Input: part model. Units: mm. Frame: model coordinates. A direction names the side the tool comes from. Coordinates: 2 decimals unless noted, no trailing zeros. Write each loop counter-clockwise with the first axis right and the second up, starting at its lowest first coordinate (ties: lowest second). Pieces come first, ordered by that corner, then holes. Notation, with made-up numbers: (-6, 72.25) - (39, 72.25) arc R33 cw to (39, 104.25) - close; hole circle Ø4 at (17.25, 74). An arc over 180 degrees is marked (long way). One line per question, with ' | ' between items. Start each with the question number.
1) First-contact query: P1, Ø1, axis at y = -11, z = 15.5, coming from the -X side; P2, Ø8, axis at x = -27.5, y = -16.5, coming from the -Z side; P3, Ø3.5, axis at x = -32, y = -14.5, coming from the +Z side; P4, Ø10, axis at x = -31, y = 25, coming from the -Z side. Flat tips, straight axial feed; report the tip coordinate or a pass-through.
2) Section query A-A on x = -25. Return loops of the section in (y, z), and give its area (3 significant figures).
3) Section query B-B on y = -15. Return loops of the section in (x, z), and give its area (3 significant figures).
4) Line query: line 1 (X direction, y = -9, z = 19.75); line 2 (X direction, y = 17.5, z = 12); line 3 (X direction, y = -14.5, z = 8.5). Output: solid intervals per line, ascending.
5) Reachability of faces 1 (the flat face through (-30, -15, 7.621)), 2 (the flat face through (-35.132, -15, 13)), 3 (the flat face through (-30, -15, 19.284)), 4 (the flat face through (-22.931, 31, 13)) from +Z, -Z, +X, -X, +Y, -Y: full face, straight path, thin tool, end or side. Return the list, or none.
6) Section query C-C on x = -33.5. Return loops of the section in (y, z).
7) Section query D-D on y = -5. Return loops of the section in (x, z).
```python
from build123d import *

# Parameters (mm, degrees)
F1_DEPTH = 25.4
F3_W     = 10.9566785395
F3_H     = 11.6627290845
F4_DEPTH = 7.1539785713


with BuildPart() as f1:
    # F0 (on Top) → F1 (new body)
    with BuildSketch(Plane.XY):
        with BuildLine():
            Line((-42.3919206649, 8.6023595556), (-42.3919206649, -11.4512224138))
            Line((-42.3919206649, -11.4512224138), (-19.3287206649, -11.4512224138))
            Line((-19.3287206649, -11.4512224138), (-19.3287206649, 8.6023595556))
            add(Edge.make_bspline(
                [(-19.3287206649, 8.6023595556), (-16.323673708, 11.7888919971), (-9.9481352571, 18.5494707236), (-16.0846098572, 27.4246591557), (-19.3287206649, 32.1166146935)],
                knots=[0, 0, 0, 0, 0.4713400446, 1, 1, 1, 1], degree=3))
            Line((-19.3287206649, 32.1166146935), (-22.9309096968, 32.1166146935))
            Line((-22.9309096968, 32.1166146935), (-22.9309096968, 29.055005683))
            ThreePointArc((-22.9309096968, 29.055005683), (-30.8603206649, 11.9618341392), (-38.7897316331, 29.055005683))
            Line((-38.7897316331, 29.055005683), (-38.7897316331, 32.1166146935))
            Line((-38.7897316331, 32.1166146935), (-42.3919206649, 32.1166146935))
            add(Edge.make_bspline(
                [(-42.3919206649, 8.6023595556), (-45.3969676218, 11.7888919971), (-51.7725060727, 18.5494707236), (-45.6360314726, 27.4246591557), (-42.3919206649, 32.1166146935)],
                knots=[0, 0, 0, 0, 0.4713400446, 1, 1, 1, 1], degree=3))
        make_face()
    extrude(amount=F1_DEPTH)

    # F3 (on face) → F4 (join)
    with BuildSketch(Plane.XZ.offset(11.4512224138)):
        with Locations((-29.654065147, 13.45269382)):
            Rectangle(F3_W, F3_H)
    extrude(amount=F4_DEPTH)


solid = f1.part
```
Answer key:
1) P1: x = -42.39 | P2: z = 7.62 | P3: z = 19.28 | P4: through
2) outline: (-18.61, 7.62) - (-11.45, 7.62) - (-11.45, 0) - (13.77, 0) - (13.77, 25.4) - (-11.45, 25.4) - (-11.45, 19.28) - (-18.61, 19.28) - close | area: 724 mm²
3) outline: (-35.13, 7.62) - (-24.18, 7.62) - (-24.18, 19.28) - (-35.13, 19.28) - close | area: 128 mm²
4) line 1: -42.39 to -19.33 | line 2: -48.47 to -40.05, -21.68 to -13.25 | line 3: -35.13 to -24.18
5) face 1: -Z, +X, -X, -Y | face 2: +Z, -Z, -X, -Y | face 3: +Z, +X, -X, -Y | face 4: +Z, -Z, +Y
6) outline: (-18.61, 7.62) - (-11.45, 7.62) - (-11.45, 0) - (12.3, 0) - (12.3, 25.4) - (-11.45, 25.4) - (-11.45, 19.28) - (-18.61, 19.28) - close
7) outline: (-42.39, 0) - (-19.33, 0) - (-19.33, 25.4) - (-42.39, 25.4) - close
